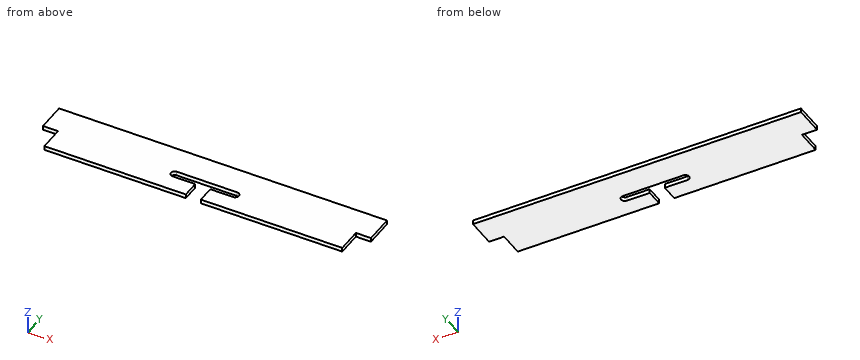
Autodesk Fusion 360 part; units mm, degrees
sketch "Sketch1" plane through (0, 0, 0) normal (0, 0, 1) x (1, 0, 0)
  line L0 (0, 0) -> (433.8, 0)
  line L1 (433.8, 0) -> (433.8, 70.4)
  line L2 (433.8, 70.4) -> (0, 70.4)
  line L3 (0, 70.4) -> (0, 0)
  line L4 (0, 0) -> (19.9, 0)
  line L5 (19.9, 0) -> (19.9, 32.4)
  line L6 (19.9, 32.4) -> (0, 32.4)
  line L7 (0, 32.4) -> (0, 0)
  line L8 (206.95, 0) -> (226.85, 0)
  line L9 (226.85, 0) -> (226.85, 32.4)
  line L10 (226.85, 32.4) -> (206.95, 32.4)
  line L11 (206.95, 32.4) -> (206.95, 0)
  line L12 (433.8, 0) -> (413.9, 0)
  line L13 (413.9, 0) -> (413.9, 32.4)
  line L14 (413.9, 32.4) -> (433.8, 32.4)
  line L15 (433.8, 32.4) -> (433.8, 0)
  dimension "d1" = 433.8
  dimension "d2" = 70.4
  dimension "d3" = 19.9
  dimension "d4" = 19.9
  dimension "d5" = 19.9
  dimension "d6" = 32.4
  dimension "d7" = 32.4
  dimension "d8" = 32.4
  dimension "d9" = 206.95
extrude "Extrude2" add sketch "Sketch1" along normal blind 5.4 contours L0 L1 L2 L3 L5 L6 L9 L10 L11 L13 L14
sketch "Sketch2" plane through (0, 0, 5.4) normal (0, 0, 1) x (1, 0, 0)
  line L0 (226.85, 0) -> (413.9, 0)
  line L1 (413.9, 0) -> (413.9, 32.4)
  line L2 (413.9, 32.4) -> (433.8, 32.4)
  line L3 (433.8, 32.4) -> (433.8, 70.4)
  line L4 (433.8, 70.4) -> (0, 70.4)
  line L5 (0, 70.4) -> (0, 32.4)
  line L6 (0, 32.4) -> (19.9, 32.4)
  line L7 (19.9, 32.4) -> (19.9, 0)
  line L8 (19.9, 0) -> (206.95, 0)
  line L9 (206.95, 0) -> (206.95, 32.4)
  line L10 (206.95, 32.4) -> (226.85, 32.4)
  line L11 (226.85, 32.4) -> (226.85, 0)
  line L12 (256.9, 32.4) -> (176.9, 32.4)
  arc A0 (176.9, 32.4) -> (176.9, 22.4) centre (176.9, 27.4) ccw
  line L13 (176.9, 22.4) -> (256.9, 22.4)
  arc A1 (256.9, 22.4) -> (256.9, 32.4) centre (256.9, 27.4) ccw
  line L14 (256.9, 27.4) -> (176.9, 27.4) construction
  point P0 (216.9, 27.4)
  dimension "d14" = 5
  dimension "d15" = 80
  dimension "d16" = 433.8
  dimension "d17" = 216.9
extrude "Extrude3" cut sketch "Sketch2" against normal blind 25 contours L11 L12 L13 A1 | L9 L12 A0 L13
sketch "export" plane through (0, 0, 5.4) normal (0, 0, 1) x (1, 0, 0)
  line L0 (206.95, 22.4) -> (176.9, 22.4)
  arc A0 (176.9, 32.4) -> (176.9, 22.4) centre (176.9, 27.4) ccw
  line L1 (176.9, 32.4) -> (256.9, 32.4)
  arc A1 (256.9, 22.4) -> (256.9, 32.4) centre (256.9, 27.4) ccw
  line L2 (256.9, 22.4) -> (226.85, 22.4)
  line L3 (226.85, 22.4) -> (226.85, 0)
  line L4 (226.85, 0) -> (413.9, 0)
  line L5 (413.9, 0) -> (413.9, 32.4)
  line L6 (413.9, 32.4) -> (433.8, 32.4)
  line L7 (433.8, 32.4) -> (433.8, 70.4)
  line L8 (433.8, 70.4) -> (0, 70.4)
  line L9 (0, 70.4) -> (0, 32.4)
  line L10 (0, 32.4) -> (19.9, 32.4)
  line L11 (19.9, 32.4) -> (19.9, 0)
  line L12 (19.9, 0) -> (206.95, 0)
  line L13 (206.95, 0) -> (206.95, 22.4)
extrude "Extrude1" [suppressed]
equation "d2 = d6 + 38 mm"
equation "d4 = d3"
equation "d5 = d4"
equation "d6 = 6 * 5.4 mm"
equation "d7 = d6"
equation "d8 = d7"
equation "d9 = ( d1 - d4 ) / 2"
equation "d17 = d16 / 2"
Model file for the job. Use its own axes, mm. Coordinates: 2 decimals unless noted, no trailing zeros. Order: outer loops, then holes, each group sorted by start corner. A loop starts at its lowest first (then second) coordinate and runs counter-clockwise, first axis right, second up. Notation, with made-up numbers: (8, 27.25) -> (57, 27.25) arc R11 cw to (57, 34.25) -> close; hole circle Ø9 at (13, 79.25). An arc over 180 degrees is marked (long way). Answer as a JSON object with one key per item and string values. Group by question number.
1) Drill centre lines: L1, parallel to X at y = 15.5, z = 1.75; L2, parallel to Y at x = 197.5, z = 4.7; L3, parallel to X at y = 28, z = 5.1. Where is each one in solid material? Low to high.
2) Cut at B-B, the plane x = 235.5. Write the cut outline in (y, z), then the cut area to 3 significant figures.
3) Flat gauge pins, fed straight in: pin 1 (2.5 mm diameter, centred on x = 214, z = 2, fed in from -Y); pin 2 (1.6 mm diameter, centred on y = 12.5, z = 2.5, fed in from -X); pin 3 (2.5 mm diameter, centred on y = 16, z = 2.5, fed in from +X). Where does each tip first touch, or does it go through?
4) Cut at A-A, the plane y = 27.4. Write the cut outline in (x, z), then the cut area to 3 significant figures.
5) Cut at C-C, the plane z = 0.9. Write the cut outline in (x, y), then the cut area to 3 significant figures.
Check values:
{
 "1": {"L1": "x = 19.9 to 206.95, 226.85 to 413.9", "L2": "y = 0 to 22.4, 32.4 to 70.4", "L3": "x = 19.9 to 171.94, 261.86 to 413.9"},
 "2": {"outline": "(0, 0) -> (22.4, 0) -> (22.4, 5.4) -> (0, 5.4) -> close; (32.4, 0) -> (70.4, 0) -> (70.4, 5.4) -> (32.4, 5.4) -> close", "area": "326 mm²"},
 "3": {"pin 1": "stops at y = 32.4", "pin 2": "stops at x = 19.9", "pin 3": "stops at x = 413.9"},
 "4": {"outline": "(19.9, 0) -> (171.9, 0) -> (171.9, 5.4) -> (19.9, 5.4) -> close; (261.9, 0) -> (413.9, 0) -> (413.9, 5.4) -> (261.9, 5.4) -> close", "area": "1,640 mm²"},
 "5": {"outline": "(0, 32.4) -> (19.9, 32.4) -> (19.9, 0) -> (206.95, 0) -> (206.95, 22.4) -> (176.9, 22.4) arc R5 cw to (176.9, 32.4) -> (256.9, 32.4) arc R5 cw to (256.9, 22.4) -> (226.85, 22.4) -> (226.85, 0) -> (413.9, 0) -> (413.9, 32.4) -> (433.8, 32.4) -> (433.8, 70.4) -> (0, 70.4) -> close", "area": "27,900 mm²"}
}
